from build123d import *

# Parameters (mm, degrees)
CUT_EXTRUDE_1_DEPTH = 2.08


with BuildPart() as part:
    # 草图1 → 旋转1 (revolve)
    with BuildSketch(Plane.XY, mode=Mode.PRIVATE) as revolve_1_sk:
        with BuildLine():
            Line((2.5, 0), (0, 0))
            Line((0, 0), (0, 28.5))
            Line((0, 28.5), (3.3, 28.5))
            ThreePointArc((3.3, 28.5), (4.466476871, 27.179336894), (5, 25.5))
            Line((5, 25.5), (5, 25))
            Line((5, 25), (3, 25))
            Line((3, 25), (2.5, 24.614874776))
            Line((2.5, 24.614874776), (3, 24.229749551))
            Line((3, 24.229749551), (2.5, 23.844624327))
            Line((2.5, 23.844624327), (3, 23.459499102))
            Line((3, 23.459499102), (2.5, 23.074373878))
            Line((2.5, 23.074373878), (3, 22.689248653))
            Line((3, 22.689248653), (2.5, 22.304123429))
            Line((2.5, 22.304123429), (3, 21.918998204))
            Line((3, 21.918998204), (2.5, 21.53387298))
            Line((2.5, 21.53387298), (3, 21.148747755))
            Line((3, 21.148747755), (2.5, 20.763622531))
            Line((2.5, 20.763622531), (3, 20.378497306))
            Line((3, 20.378497306), (2.5, 19.993372082))
            Line((2.5, 19.993372082), (3, 19.608246857))
            Line((3, 19.608246857), (2.5, 19.223121633))
            Line((2.5, 19.223121633), (3, 18.837996408))
            Line((3, 18.837996408), (2.5, 18.452871184))
            Line((2.5, 18.452871184), (3, 18.06774596))
            Line((3, 18.06774596), (2.5, 17.682620735))
            Line((2.5, 17.682620735), (3, 17.297495511))
            Line((3, 17.297495511), (2.5, 16.912370286))
            Line((2.5, 16.912370286), (3, 16.527245062))
            Line((3, 16.527245062), (2.5, 16.142119837))
            Line((2.5, 16.142119837), (3, 15.756994613))
            Line((3, 15.756994613), (2.5, 15.371869388))
            Line((2.5, 15.371869388), (3, 14.986744164))
            Line((3, 14.986744164), (2.5, 14.601618939))
            Line((2.5, 14.601618939), (3, 14.216493715))
            Line((3, 14.216493715), (2.5, 13.83136849))
            Line((2.5, 13.83136849), (3, 13.446243266))
            Line((3, 13.446243266), (2.5, 13.061118041))
            Line((2.5, 13.061118041), (3, 12.675992817))
            Line((3, 12.675992817), (2.5, 12.290867592))
            Line((2.5, 12.290867592), (3, 11.905742368))
            Line((3, 11.905742368), (2.5, 11.520617143))
            Line((2.5, 11.520617143), (3, 11.135491919))
            Line((3, 11.135491919), (2.5, 10.750366695))
            Line((2.5, 10.750366695), (3, 10.36524147))
            Line((3, 10.36524147), (2.5, 9.980116246))
            Line((2.5, 9.980116246), (3, 9.594991021))
            Line((3, 9.594991021), (2.5, 9.209865797))
            Line((2.5, 9.209865797), (3, 8.824740572))
            Line((3, 8.824740572), (2.5, 8.439615348))
            Line((2.5, 8.439615348), (3, 8.054490123))
            Line((3, 8.054490123), (2.5, 7.669364899))
            Line((2.5, 7.669364899), (3, 7.284239674))
            Line((3, 7.284239674), (2.5, 6.89911445))
            Line((2.5, 6.89911445), (3, 6.513989225))
            Line((3, 6.513989225), (2.5, 6.128864001))
            Line((2.5, 6.128864001), (3, 5.743738776))
            Line((3, 5.743738776), (2.5, 5.358613552))
            Line((2.5, 5.358613552), (3, 4.973488327))
            Line((3, 4.973488327), (2.5, 4.588363103))
            Line((2.5, 4.588363103), (3, 4.203237879))
            Line((3, 4.203237879), (2.5, 3.818112654))
            Line((2.5, 3.818112654), (3, 3.43298743))
            Line((3, 3.43298743), (2.5, 3.047862205))
            Line((2.5, 3.047862205), (3, 2.662736981))
            Line((3, 2.662736981), (2.5, 2.277611756))
            Line((2.5, 2.277611756), (3, 1.892486532))
            Line((3, 1.892486532), (2.5, 1.507361307))
            Line((2.5, 1.507361307), (3, 1.122236083))
            Line((3, 1.122236083), (2.5, 0.737110858))
            Line((2.5, 0.737110858), (2.916387895, 0.416387895))
            Line((2.916387895, 0.416387895), (2.5, 0))
        make_face()
    revolve(revolve_1_sk.sketch.rotate(Axis((0, 25.075303233, 0), (0, 1, 0)), 90), axis=Axis((0, 25.075303233, 0), (0, 1, 0)))

    # 草图3 → 切除-拉伸1 (cut)
    with BuildSketch(Plane(origin=(0, 28.5, 0), x_dir=(1, 0, 0), z_dir=(0, 1, 0))):
        Polygon((2.357898499, 0), (1.17894925, 2.042), (-1.17894925, 2.042), (-2.357898499, 0), (-1.17894925, -2.042), (1.17894925, -2.042), align=None)
    extrude(amount=-CUT_EXTRUDE_1_DEPTH, mode=Mode.SUBTRACT)


solid = part.part
Source: CAD feature listing. Evaluate the final solid. Frame: model axes, mm. A direction names the side the tool comes from. Give positions to 0.01 mm unless a question says otherwise; leave off trailing zeros. Write item = value, one per line.
Q1. Line query: line 1 (Y direction, x = -0.5, z = 0); line 2 (Z direction, x = 1, y = 6.75); line 3 (Z direction, x = 2.25, y = 27.25). Output: solid intervals per line, ascending. Write a range as from..to.
Here are the results:
line_1 = 0..26.42
line_2 = -2.5..2.5
line_3 = -3.81..-0.19, 0.19..3.81
Q2. Reachability of faces 1 (the face through (0, 27, -2.042)), 2 (the face through (-0.22, 25.246, 4.995)) from +Z, -Z, +X, -X, +Y, -Y: full face, straight path, thin tool, end or side. Return the list, or none.
Here are the results:
face_1 = +Y
face_2 = +Y, -Y
Q3. First-contact query: pin 1 (2.5 mm diameter, centred on x = 0.5, y = 27.5, fed in from -Z); pin 2 (2 mm diameter, centred on x = -3.5, z = -3, fed in from +Y); pin 3 (1 mm diameter, centred on x = -0.5, y = 27.5, fed in from +Z). Flat tips, straight axial feed; report the tip coordinate or a pass-through.
Here are the results:
pin_1 = -4.84
pin_2 = 28.25
pin_3 = 4.54
